from build123d import *

# Parameters (mm, degrees)
BOSS_EXTRUDE1_DEPTH = 6.35
SKETCH1_4_W         = 6.35
SKETCH1_4_H         = 6.35
BOSS_EXTRUDE2_DEPTH = 6.35


with BuildPart() as part:
    # Sketch1 → Boss-Extrude1 (new body)
    with BuildSketch(Plane(origin=(0, 0, 0), x_dir=(0, 0, -1), z_dir=(1, 0, 0))):
        Polygon((-76.2, 25.4), (-76.2, 12.7), (-69.85, 12.7), (-69.85, 0), (-76.2, 0), (-76.2, -12.7), (-69.85, -12.7), (-69.85, -31.75), (-63.5, -31.75), (-63.5, -25.4), (-38.1, -25.4), (-38.1, -31.75), (-31.75, -31.75), (-31.75, -25.4), (31.75, -25.4), (31.75, -31.75), (38.1, -31.75), (38.1, -25.4), (63.5, -25.4), (63.5, -31.75), (69.85, -31.75), (69.85, -25.4), (76.2, -25.4), (76.2, -12.7), (69.85, -12.7), (69.85, 0), (76.2, 0), (76.2, 12.7), (69.85, 12.7), (69.85, 25.4), (19.05, 25.4), (19.05, 12.7), (-19.05, 12.7), (-19.05, 25.4), align=None)
    extrude(amount=BOSS_EXTRUDE1_DEPTH)

    # Sketch1<4> → Boss-Extrude2 (add)
    with BuildSketch(Plane(origin=(0, 0, 0), x_dir=(0, 0, -1), z_dir=(1, 0, 0))):
        with Locations((73.025, -28.575)):
            Rectangle(SKETCH1_4_W, SKETCH1_4_H)
    extrude(amount=BOSS_EXTRUDE2_DEPTH)


solid = part.part
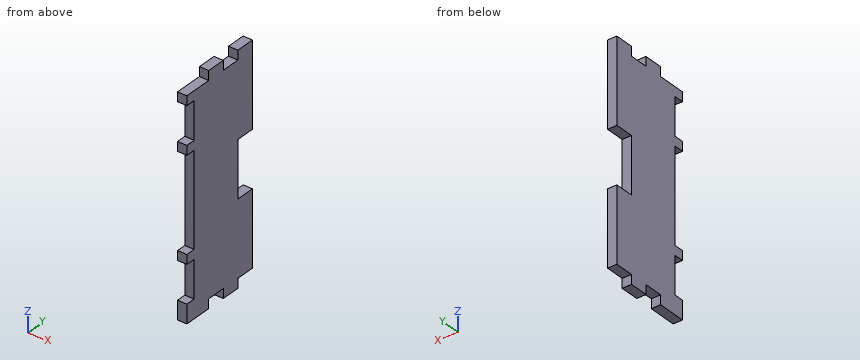
Can you work these out from the model? Positions are in its coordinate system, mm. Round coordinates to 2 decimals unless told otherwise and drop trailing zeros. Write each loop counter-clockwise with the first axis right and the second up, starting at its lowest first coordinate (ties: lowest second). Pieces come first, ordered by that corner, then holes. Notation, with made-up numbers: (-14.5, 5.25) - (13.5, 5.25) arc R31 ccw to (13.5, 41.25) - close; hole circle Ø1 at (82.5, -32.5). An arc over 180 degrees is marked (long way). Write each question's results on one line, items separated by ' | '. Start each with the question number.
1) Please list where these lines run through material, in increasing order: line 1 (Z direction, x = 4.25, y = -26); line 2 (Z direction, x = 5.25, y = 13.5); line 3 (Y direction, x = 1.75, z = 58.5).
2) For pin 1 Ø3 at (x, y) = (2, -8.5) entering from -Z; pin 2 Ø1 at (x, y) = (2.5, 7) entering from +Z; pin 3 Ø1.9 at (x, z) = (4.5, -74.5) entering from +Y, each with a flat end and sliding along its axis, tell me the tip position at first contact or that it passes through.
3) Suppose I cut it at A-A (y = 21.5). List the corners of the cut face in (x, z) for me.
4) Suppose I cut it at B-B (y = -27). List the corners of the cut face in (x, z) for me.
5) Suppose I cut it at D-D (z = -4). List the corners of the cut face in (x, y) for me.
Here are the results:
1) line 1: z = -76.2 to -63.5, -38.1 to -31.75, 31.75 to 38.1, 63.5 to 69.85 | line 2: z = -69.85 to -19.05, 19.05 to 76.2 | line 3: y = -25.4 to 25.4
2) pin 1: stops at z = -69.85 | pin 2: stops at z = 69.85 | pin 3: stops at y = 12.7
3) outline: (0, -69.85) - (6.35, -69.85) - (6.35, -19.05) - (0, -19.05) - close; (0, 19.05) - (6.35, 19.05) - (6.35, 76.2) - (0, 76.2) - close
4) outline: (0, -76.2) - (6.35, -76.2) - (6.35, -63.5) - (0, -63.5) - close; (0, -38.1) - (6.35, -38.1) - (6.35, -31.75) - (0, -31.75) - close; (0, 31.75) - (6.35, 31.75) - (6.35, 38.1) - (0, 38.1) - close; (0, 63.5) - (6.35, 63.5) - (6.35, 69.85) - (0, 69.85) - close
5) outline: (0, -25.4) - (6.35, -25.4) - (6.35, 12.7) - (0, 12.7) - close
